Job drawing, mm, ordinate dimensions from the low corner. One solid piece. A direction names the side the tool comes from. Round coordinates to 2 decimals unless told otherwise and drop trailing zeros. Loops run counter-clockwise (first coordinate to the right, second up) from the corner with the lowest first, then second, coordinate; pieces in that order, holes last.
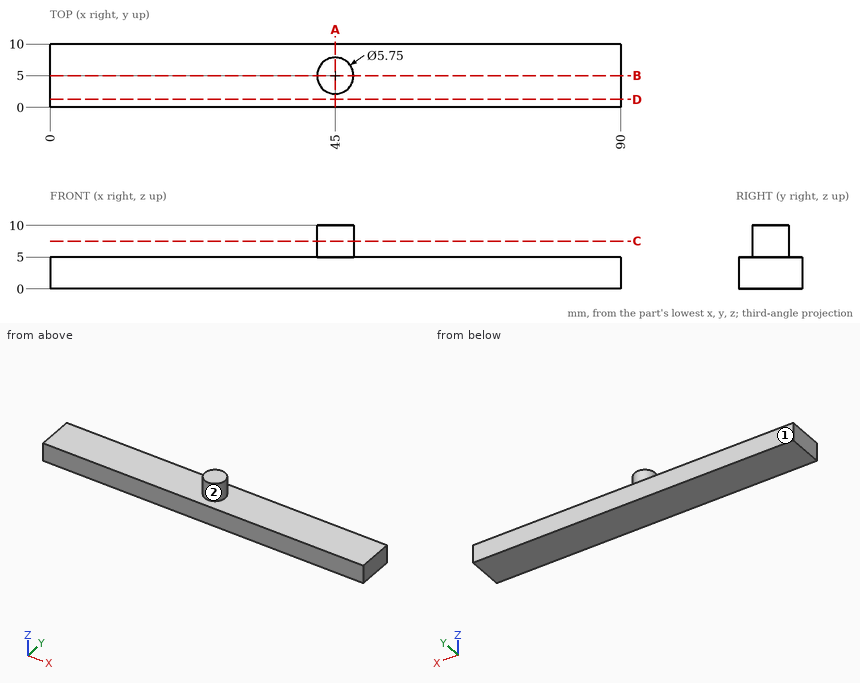
1) Tool access for the marked faces 1 and 2: list every direction of +Z, -Z, +X, -X, +Y, -Y with a clear straight run to the whole face (end or side of a thin tool).
Values:
face 1: +Z, -Z, +X, -X, +Y
face 2: +Z
2) Wall check: line 1 along Z through (x, y) = (19, 5.75); line 2 along X through (y, z) = (3.5, 6.75); line 3 along X through (y, z) = (6.75, 6.5). Give the ranges that are in metal, low to high.
Values:
line 1: z = 0 to 5
line 2: x = 42.55 to 47.45
line 3: x = 42.72 to 47.28
3) Slice it at D-D, the plane y = 1.25. Give the cut face in (x, z), then the cut area to 3 significant figures.
Values:
outline: (0, 0) - (90, 0) - (90, 5) - (0, 5) - close
area: 450 mm2
4) Drop flat-ended pins along their axis: pin 1 Ø6 at (y, z) = (8.5, 8.5) entering from +X; pin 2 Ø3 at (x, y) = (53.5, 7) entering from +Z. Give the stop position or say it passes through.
Values:
pin 1: stops at x = 47.83
pin 2: stops at z = 5
5) Slice it at A-A, the plane x = 45. Give the cut face in (y, z) (3 decimals), then the cut area to 4 significant figures.
Values:
outline: (0, 0) - (10, 0) - (10, 5) - (7.875, 5) - (7.875, 10) - (2.125, 10) - (2.125, 5) - (0, 5) - close
area: 78.75 mm2
6) Slice it at C-C, the plane z = 7.5. Give the cut face in (x, y) (3 decimals), then the cut area to 3 significant figures.
Values:
outline: circle Ø5.75 at (45, 5)
area: 26.0 mm2
7) Slice it at B-B, the plane y = 5. Give the cut face in (x, z) (3 decimals), then the cut area to 3 significant figures.
Values:
outline: (0, 0) - (90, 0) - (90, 5) - (47.875, 5) - (47.875, 10) - (42.125, 10) - (42.125, 5) - (0, 5) - close
area: 479 mm2
